```python
from build123d import *

# Parameters (mm, degrees)
F2_R    = 6.5
F3_SIZE = 2


with BuildPart() as f1:
    # F0 (on Top) → F1 (revolve)
    with BuildSketch(Plane.XY):
        Polygon((-74.077871, 8.5), (-74.077871, 3.673849), (-44.077871, 3.673849), (-41.102886, 1), (-39.102886, 1), (-39.102886, 9), (-59.077871, 10), (-59.077871, 8.5), align=None)
    revolve(axis=Axis((5.52991, 0, 0), (1, 0, 0)))

    # F2
    f2_edges = [f1.edges().sort_by_distance(p)[0] for p in [
        (-39.102886, -9, 0),
    ]]
    fillet(f2_edges, radius=F2_R)

    # F3
    f3_edges = [f1.edges().sort_by_distance(p)[0] for p in [
        (-74.077871, -3.673849, 0),
    ]]
    chamfer(f3_edges, length=F3_SIZE)


solid = f1.part
```
For this review, take the finished solid that the model builds, in its own axes (mm). A direction names the side the tool comes from. Coordinates: 2 decimals unless noted, no trailing zeros. Write each loop counter-clockwise with the first axis right and the second up, starting at its lowest first coordinate (ties: lowest second). Pieces come first, ordered by that corner, then holes. Notation, with made-up numbers: (55.25, 65) - (83.25, 65) arc R6 cw to (83.25, 74) - close; hole circle Ø5 at (78, 19). An arc over 180 degrees is marked (long way). Answer in a Markdown table with one row per item. Add a question column.
Q1. We need section B-B, the plane x = -50. State the section outline as (y, z) points, and give its area (3 significant figures).
Q2. For probe 1 along Y at (x, z) = (-59, -1.5); probe 2 along Z at (x, y) = (-40.25, 0); probe 3 along Z at (x, y) = (-71.5, -3), list the stretches that pass through material, from the lowest coordinate up.
Q3. We need section A-A, the plane x = -46. State the section outline as (y, z) points.
Q4. Draft analysis for pull direction Z (two halves, no side actions). For faces 3 (the cylindrical face through (-66.683, 4.57, 7.167)), 4 (the conical face through (-72.2, 3.62, 1.14)), 5 (the flat face through (-59.078, -4.5, -7.4)), state which applies: +Z half, -Z half, draft (parallel to the pull), parting line (faces both ways), or undercut.
Q5. For P1, Ø8, axis at x = -53.5, y = -4, coming from the -Z side; P2, Ø5, axis at x = -51.5, z = -6.5, coming from the +Y side; P3, Ø1, axis at x = -63.5, y = -4.5, coming from the +Z side, all flat-tipped, find the tip position at first contact; note any pin that passes through.
Q6. Tool access review of faces 1 (the cylindrical face through (-57.882, 1.975, 3.098)), 2 (the flat face through (-74.078, 2, -6)): name each direction out of +Z, -Z, +X, -X, +Y, -Y from which nothing blocks a thin tool from reaching the whole face with its end or side.
Answer list:
| question | item | result |
|---|---|---|
| 1 | outline | circle Ø19.09 at (0, 0); hole circle Ø7.35 at (0, 0) |
| 1 | area | 244 mm2 |
| 2 | probe 1 | y = -9.88 to -3.35, 3.35 to 9.88 |
| 2 | probe 2 | z = -6.5 to -1, 1 to 6.5 |
| 2 | probe 3 | z = -7.95 to -2.12, 2.12 to 7.95 |
| 3 | outline | circle Ø18.69 at (0, 0); hole circle Ø7.35 at (0, 0) |
| 4 | face 3 | parting line |
| 4 | face 4 | undercut |
| 4 | face 5 | draft |
| 5 | P1 | stops at z = -9.81 |
| 5 | P2 | stops at y = 8.76 |
| 5 | P3 | stops at z = 7.5 |
| 6 | face 1 | -X |
| 6 | face 2 | +Z, -Z, -X, +Y, -Y |
